Part print with two shaded views. Sizes in mm from the minimum x, y, z corner. Round coordinates to 2 decimals unless told otherwise and drop trailing zeros. Write each loop counter-clockwise with the first axis right and the second up, starting at its lowest first coordinate (ties: lowest second). Pieces come first, ordered by that corner, then holes. Notation, with made-up numbers: M 24.5,30 L 46.5,30 A23 cw 46.5,43 Z; hole C 0.25,1.25 d3. An arc over 180 degrees is marked long. One line per question, with ' | ' between items. Start each with the question number.
1) Drop a flat-ended pin along its axis: pin 1 Ø1.5 at (x, z) = (5.5, 61) entering from -Y. Give the stop position or say it passes through.
2) Wall check: probe 1 along Z at (x, y) = (1.25, 73); probe 2 along Y at (x, z) = (0.5, 4.5); probe 3 along Z at (x, y) = (1, 13.5). Give the ranges that are in metal, low to high. Write a range as [from, to].
3) Saw through at B-B (y = 16). List the corners of the cut face in (x, z) (3 decimals).
4) Saw through at C-C (z = 35). List the corners of the cut face in (x, y).
5) Saw through at A-A (x = 3.5). List the corners of the cut face in (y, z) (3 decimals), plus the area to 3 significant figures.
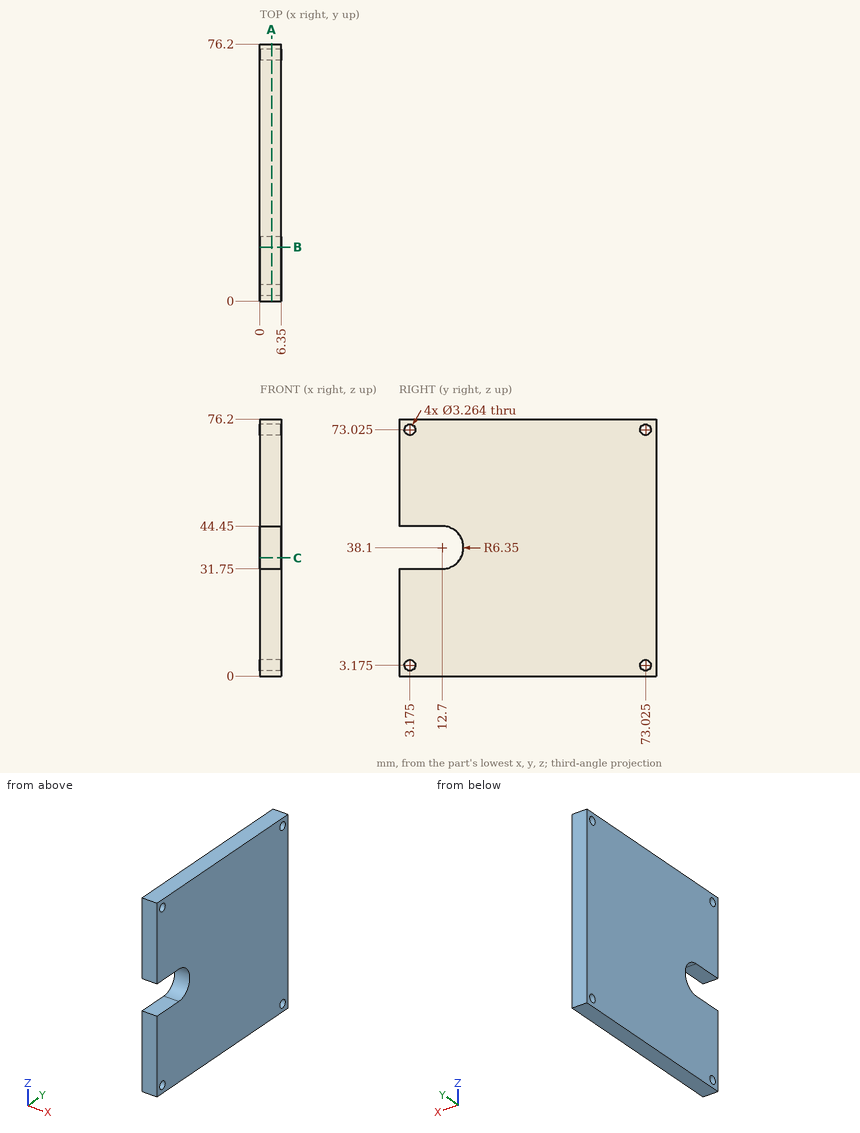
Answer key:
1) pin 1: stops at y = 0
2) probe 1: z = [0, 1.54], [4.81, 71.39], [74.66, 76.2] | probe 2: y = [0, 2.22], [4.13, 72.07], [73.98, 76.2] | probe 3: z = [0, 31.8], [44.4, 76.2]
3) outline: M 0,0 L 6.35,0 L 6.35,32.675 L 0,32.675 Z; M 0,43.525 L 6.35,43.525 L 6.35,76.2 L 0,76.2 Z
4) outline: M 0,18.24 L 6.35,18.24 L 6.35,76.2 L 0,76.2 Z
5) outline: M 0,0 L 76.2,0 L 76.2,76.2 L 0,76.2 L 0,44.45 L 12.7,44.45 A6.35 cw 12.7,31.75 L 0,31.75 Z; hole C 3.175,3.175 d3.264; hole C 3.175,73.025 d3.264; hole C 73.025,3.175 d3.264; hole C 73.025,73.025 d3.264 | area: 5,550 mm2
